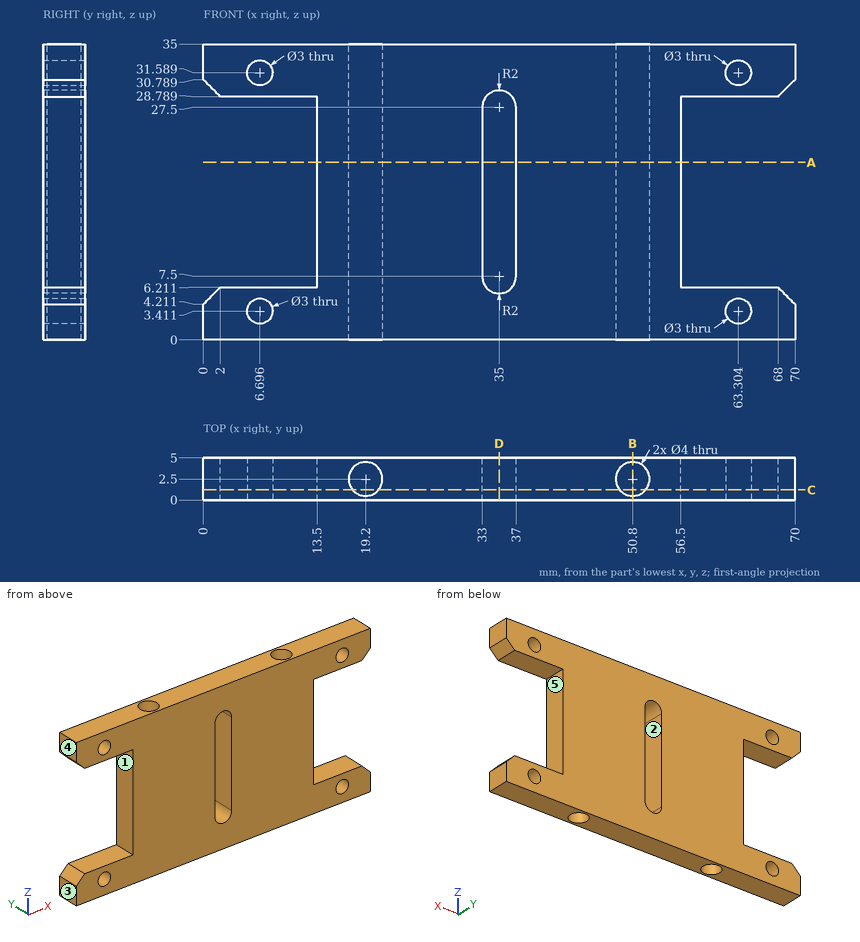
For this review, use the dimensioned drawing (mm, ordinates from the lowest corner) and the shaded views. A direction names the side the tool comes from. Give positions to 0.01 mm unless a question says otherwise; leave off trailing zeros. Write each loop counter-clockwise with the first axis right and the second up, starting at its lowest first coordinate (ties: lowest second). Pieces come first, ordered by that corner, then holes. Notation, with made-up numbers: M 68,86.5 L 73,86.5 A21 cw 73,105.5 Z; hole C 69.5,27.5 d4. An arc over 180 degrees is marked long. Answer as a JSON object with one key per item and string values. Group by question number.
1) For line 1 along Z through (x, y) = (63.5, 4.4) (1 decimal); line 2 along Z through (x, y) = (4, 4.2); line 3 along X through (y, z) = (2.6, 4.5) (1 decimal), list the stretches that pass through material, from the lowest coordinate up.
2) We need section D-D (x = 35). Give the boundary of the cut face in (y, z), and give its area (3 significant figures).
3) We need section C-C (y = 1.2). Count the separate pieces of the cut face and the enclosed holes in it, and give its area (3 significant figures).
4) Tool access review of the marked faces 1, 2 and 3: name each direction out of +Z, -Z, +X, -X, +Y, -Y from which nothing blocks a thin tool from reaching the whole face with its end or side.
5) We need section A-A (z = 21). Give the boundary of the cut face in (x, y).
6) Clearance check with flat-ended pins moving along their axes: pin 1 Ø2.5 at (x, z) = (63.3, 3.41) entering from -Y; pin 2 Ø2.5 at (y, z) = (2.5, 20.5) entering from -X; pin 3 Ø2 at (y, z) = (3.5, 14.5) entering from +X. State where each tip first meets the part, or that it passes through.
7) We need section B-B (x = 50.8). Give the boundary of the cut face in (y, z).
8) Mouldability with a two-part tool opening along Z and no side actions: class the marked faces 4 and 5 as released by +Z, released by -Z, zero draft, split by the parting line, or undercut.
Answer key:
{
 "1": {"line 1": "z = 0 to 1.9, 4.9 to 6.2, 28.8 to 30.1, 33.1 to 35", "line 2": "z = 0 to 6.21, 28.79 to 35", "line 3": "x = 0.3 to 5.7, 7.7 to 17.2, 21.2 to 48.8, 52.8 to 62.3, 64.3 to 69.7"},
 "2": {"outline": "M 0,0 L 5,0 L 5,5.5 L 0,5.5 Z; M 0,29.5 L 5,29.5 L 5,35 L 0,35 Z", "area": "55.0 mm²"},
 "3": {"separate pieces": "3", "enclosed holes": "5", "area": "1,500 mm²"},
 "4": {"face 1": "-X, +Y, -Y", "face 2": "+Y, -Y", "face 3": "+Z, -Z, -X, +Y, -Y"},
 "5": {"outline": "M 13.5,0 L 33,0 L 33,5 L 13.5,5 Z; M 37,0 L 56.5,0 L 56.5,5 L 37,5 Z; hole C 19.2,2.5 d4; hole C 50.8,2.5 d4"},
 "6": {"pin 1": "passes through", "pin 2": "stops at x = 13.5", "pin 3": "stops at x = 56.5"},
 "7": {"outline": "M 0,0 L 0.5,0 L 0.5,35 L 0,35 Z; M 4.5,0 L 5,0 L 5,35 L 4.5,35 Z"},
 "8": {"face 4": "zero draft", "face 5": "undercut"}
}
